Design review of the part built by this model. Coordinates are the model's own, in mm. A direction names the side the tool comes from. Round coordinates to 2 decimals unless told otherwise and drop trailing zeros. Order: outer loops, then holes, each group sorted by start corner. A loop starts at its lowest first (then second) coordinate and runs counter-clockwise, first axis right, second up. Notation, with made-up numbers: (-27.75, 2.25) - (-0.75, 2.25) arc R12 cw to (-0.75, 14.25) - close; hole circle Ø4 at (69, -16.5). An arc over 180 degrees is marked (long way). Answer as a JSON object with one key per item and string values. Group by question number.
from build123d import *

# Parameters (mm, degrees)
SKETCH1_W           = 72.6
SKETCH1_H           = 35.5
BOSS_EXTRUDE1_DEPTH = 27
FILLET1_R           = 10
SKETCH2_W           = 52.4
SKETCH2_H           = 8
BOSS_EXTRUDE2_DEPTH = 0.1
SKETCH3_W           = 50.8
SKETCH3_H           = 18.9
BOSS_EXTRUDE3_DEPTH = 0.1
BOSS_EXTRUDE4_DEPTH = 0.2
SKETCH5_W           = 53.5
SKETCH5_H           = 19.7
BOSS_EXTRUDE5_DEPTH = 0.1


with BuildPart() as part:
    # Sketch1 → Boss-Extrude1 (new body)
    with BuildSketch(Plane.XY):
        Rectangle(SKETCH1_W, SKETCH1_H)
    extrude(amount=BOSS_EXTRUDE1_DEPTH)

    # Fillet1
    fillet1_edges = [part.edges().sort_by_distance(p)[0] for p in [
        (-36.3, 0, 27),
        (-36.3, 0, 0),
    ]]
    fillet(fillet1_edges, radius=FILLET1_R)

    # Sketch2 → Boss-Extrude2 (add)
    with BuildSketch(Plane(origin=(0, 17.75, 0), x_dir=(1, 0, 0), z_dir=(0, 1, 0))):
        with Locations((9.1, -5)):
            Rectangle(SKETCH2_W, SKETCH2_H)
        with Locations((9.1, -13.5)):
            Rectangle(SKETCH2_W, SKETCH2_H)
        with Locations((9.1, -22)):
            Rectangle(SKETCH2_W, SKETCH2_H)
    extrude(amount=BOSS_EXTRUDE2_DEPTH)

    # Sketch3 → Boss-Extrude3 (add)
    with BuildSketch(Plane.XY.offset(27)):
        with Locations((7.1, 0.25)):
            Rectangle(SKETCH3_W, SKETCH3_H)
    extrude(amount=BOSS_EXTRUDE3_DEPTH)

    # Sketch4 → Boss-Extrude4 (add)
    with BuildSketch(Plane(origin=(0, 17.75, 0), x_dir=(1, 0, 0), z_dir=(0, 1, 0))):
        with BuildLine():
            Line((-26.3, 0), (-17.1, 0))
            Line((-17.1, 0), (-17.1, -27))
            Line((-17.1, -27), (-26.3, -27))
            ThreePointArc((-26.3, -27), (-33.371067812, -24.071067812), (-36.3, -17))
            Line((-36.3, -17), (-36.3, -10))
            ThreePointArc((-36.3, -10), (-33.371067812, -2.928932188), (-26.3, 0))
        make_face()
    extrude(amount=BOSS_EXTRUDE4_DEPTH)

    # Sketch5 → Boss-Extrude5 (add)
    with BuildSketch(Plane(origin=(0, 0, 0), x_dir=(-1, 0, 0), z_dir=(0, 0, -1))):
        with Locations((-6.524728086, 1.45)):
            Rectangle(SKETCH5_W, SKETCH5_H)
    extrude(amount=BOSS_EXTRUDE5_DEPTH)


solid = part.part
1. To check wall thickness, follow line 1 (Y direction, x = -2, z = 2); line 2 (Z direction, x = -22, y = -3); line 3 (Z direction, x = 20, y = 11). State the ranges of each line that lie inside material, in increasing order. Write a range as from..to.
2. Tool access review of faces 1 (the flat face through (9, 17.85, 22)), 2 (the flat face through (-36.3, 0, 14)): name each direction out of +Z, -Z, +X, -X, +Y, -Y from which nothing blocks a thin tool from reaching the whole face with its end or side.
3. Take a section at C-C, the plane x = -30. Give the boundary of the cut face in (y, z), then the cut area to 3 significant figures.
4. Take a section at D-D, the plane y = -10. Give the boundary of the cut face in (x, z), then the cut area to 3 significant figures.
5. Take a section at B-B, the plane z = 22.5. Give the boundary of the cut face in (x, y).
6. Take a section at A-A, the plane y = 7.5. Give the boundary of the cut face in (x, z), then the cut area to 3 significant figures.
7. Clearance check with flat-ended pins moving along their axes: P1, Ø3, axis at x = 9.5, z = 10, coming from the +Y side; P2, Ø6, axis at x = -29, y = 12.5, coming from the +Z side. State where each tip first meets the part, or that it passes through.
Response values:
{
 "1": {"line 1": "-17.75..17.85", "line 2": "0..27", "line 3": "-0.1..27"},
 "2": {"face 1": "+Z, -Z, +X, +Y", "face 2": "+Z, -Z, -X, +Y, -Y"},
 "3": {"outline": "(-17.75, 0.71) - (17.95, 0.71) - (17.95, 26.29) - (-17.75, 26.29) - close", "area": "913 mm2"},
 "4": {"outline": "(-36.3, 10) arc R10 ccw to (-26.3, 0) - (36.3, 0) - (36.3, 27) - (-26.3, 27) arc R10 ccw to (-36.3, 17) - close", "area": "1,920 mm2"},
 "5": {"outline": "(-34.65, -17.75) - (36.3, -17.75) - (36.3, 17.75) - (35.3, 17.75) - (35.3, 17.85) - (-17.1, 17.85) - (-17.1, 17.95) - (-34.65, 17.95) - close"},
 "6": {"outline": "(-36.3, 10) arc R10 ccw to (-26.3, 0) - (-20.23, 0) - (-20.23, -0.1) - (33.27, -0.1) - (33.27, 0) - (36.3, 0) - (36.3, 27) - (32.5, 27) - (32.5, 27.1) - (-18.3, 27.1) - (-18.3, 27) - (-26.3, 27) arc R10 ccw to (-36.3, 17) - close", "area": "1,930 mm2"},
 "7": {"P1": "y = 17.85", "P2": "z = 27"}
}
